```python
from build123d import *

# Parameters (mm, degrees)
F1_DEPTH = 25.4


with BuildPart() as f1:
    # F0 (on Top) → F1 (new body)
    with BuildSketch(Plane.XY):
        Polygon((123.5442494553, -9.8546108769), (0, 201.9159130813), (-122.2657690137, -9.8546108769), align=None)
        with BuildLine():
            Line((-4.8778088885, 178.2273002568), (0, 186.6759130813))
            Line((0, 186.6759130813), (4.8778088885, 178.2273002568))
            Line((4.8778088885, 178.2273002568), (107.7773886687, 0))
            Line((107.7773886687, 0), (14.1198557448, 0))
            ThreePointArc((14.1198557448, 0), (9.5256601261, -0.8879425347), (4.8778088885, -1.4288253328))
            ThreePointArc((4.8778088885, -1.4288253328), (-4.6759216184, -1.4443391195), (-14.1198557448, 0))
            Line((-14.1198557448, 0), (-107.7773886687, 0))
            Line((-107.7773886687, 0), (-4.8778088885, 178.2273002568))
        make_face(mode=Mode.SUBTRACT)
        with BuildLine():
            Line((-4.8778088885, 114.1285764535), (-4.8778088885, 122.8822744628))
            ThreePointArc((-4.8778088885, 122.8822744628), (-62.1710636846, 65.4026461834), (-14.1198557448, 0))
            Line((-14.1198557448, 0), (-4.8778088885, 0))
            Line((-4.8778088885, 0), (-4.8778088885, 7.3248726765))
            ThreePointArc((-4.8778088885, 7.3248726765), (-53.6241625079, 60.726724565), (-4.8778088885, 114.1285764535))
        make_face()
        with BuildLine():
            ThreePointArc((62.346655104, 60.726724565), (45.7778356363, 103.052782344), (4.8778088885, 122.8822744628))
            Line((4.8778088885, 122.8822744628), (4.8778088885, 114.1285764535))
            ThreePointArc((4.8778088885, 114.1285764535), (39.6050452669, 96.8790577412), (53.6241625079, 60.726724565))
            ThreePointArc((53.6241625079, 60.726724565), (39.6050452669, 24.5743913889), (4.8778088885, 7.3248726765))
            Line((4.8778088885, 7.3248726765), (4.8778088885, 0))
            Line((4.8778088885, 0), (14.1198557448, 0))
            ThreePointArc((14.1198557448, 0), (48.8233098985, 21.9531534991), (62.346655104, 60.726724565))
        make_face()
        with BuildLine():
            ThreePointArc((4.8778088885, 114.1285764535), (0, 114.3508870729), (-4.8778088885, 114.1285764535))
            Line((-4.8778088885, 114.1285764535), (-4.8778088885, 7.3248726765))
            ThreePointArc((-4.8778088885, 7.3248726765), (0, 7.1025620571), (4.8778088885, 7.3248726765))
            Line((4.8778088885, 7.3248726765), (4.8778088885, 114.1285764535))
        make_face()
        with BuildLine():
            Line((4.8778088885, 178.2273002568), (0, 186.6759130813))
            Line((0, 186.6759130813), (-4.8778088885, 178.2273002568))
            Line((-4.8778088885, 178.2273002568), (-4.8778088885, 122.8822744628))
            ThreePointArc((-4.8778088885, 122.8822744628), (0, 123.073379669), (4.8778088885, 122.8822744628))
            Line((4.8778088885, 122.8822744628), (4.8778088885, 178.2273002568))
        make_face()
        with BuildLine():
            ThreePointArc((4.8778088885, 122.8822744628), (0, 123.073379669), (-4.8778088885, 122.8822744628))
            Line((-4.8778088885, 122.8822744628), (-4.8778088885, 114.1285764535))
            ThreePointArc((-4.8778088885, 114.1285764535), (0, 114.3508870729), (4.8778088885, 114.1285764535))
            Line((4.8778088885, 114.1285764535), (4.8778088885, 122.8822744628))
        make_face()
        with BuildLine():
            Line((-4.8778088885, 7.3248726765), (-4.8778088885, 0))
            Line((-4.8778088885, 0), (4.8778088885, 0))
            Line((4.8778088885, 0), (4.8778088885, 7.3248726765))
            ThreePointArc((4.8778088885, 7.3248726765), (0, 7.1025620571), (-4.8778088885, 7.3248726765))
        make_face()
        with BuildLine():
            Line((-4.8778088885, 0), (-14.1198557448, 0))
            ThreePointArc((-14.1198557448, 0), (-4.6759216184, -1.4443391195), (4.8778088885, -1.4288253328))
            Line((4.8778088885, -1.4288253328), (4.8778088885, 0))
            Line((4.8778088885, 0), (-4.8778088885, 0))
        make_face()
        with BuildLine():
            ThreePointArc((4.8778088885, -1.4288253328), (9.5256601261, -0.8879425347), (14.1198557448, 0))
            Line((14.1198557448, 0), (4.8778088885, 0))
            Line((4.8778088885, 0), (4.8778088885, -1.4288253328))
        make_face()
    extrude(amount=F1_DEPTH)


solid = f1.part
```
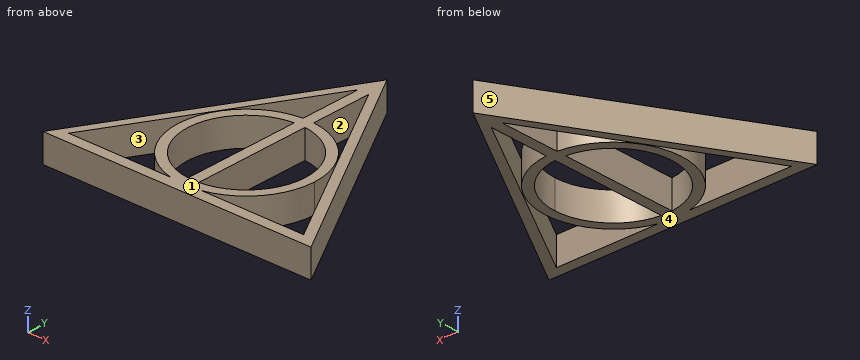
CAD build for the part. Positions are in the model's coordinates, mm. Face numbers are marked on the shaded views. A direction names the side the tool comes from. Round coordinates to 2 decimals unless told otherwise and drop trailing zeros. Order: outer loops, then holes, each group sorted by start corner. A loop starts at its lowest first (then second) coordinate and runs counter-clockwise, first axis right, second up. Notation, with made-up numbers: (61.5, 78.5) - (97.5, 78.5) arc R10 cw to (97.5, 85.5) - close; hole circle Ø5 at (76, 88.5). An arc over 180 degrees is marked (long way). Answer as CSV lines item,"result". Start each with the question number.
1. Saw through at C-C, the plane x = 74. Write the cut outline in (y, z), and give its area (3 significant figures).
2. Tool access for the marked faces 1 and 2: list every direction of +Z, -Z, +X, -X, +Y, -Y with a clear straight run to the whole face (end or side of a thin tool).
3. Saw through at A-A, the plane z = 10.25. Write the cut outline in (x, y), and give its area (3 significant figures).
4. Saw through at D-D, the plane x = -58. Write the cut outline in (y, z).
5. Drill centre lines: L1, parallel to Y at x = 34, z = 13.5; L2, parallel to X at y = 23.5, z = 16.75; L3, parallel to X at y = 150.5, z = 4 (3 decimals). Where is each one in solid material? Low to high. Write a range as [from, to].
6. Pull direction X, two halves, no side cores. Call the marked faces 3, 4 and 5: +X half, -X half, draft (parallel to the pull), parting line (faces both ways), or undercut.
7. Saw through at B-B, the plane y = 40. Write the cut outline in (x, z).
8. Pin check, flat tips, straight feed: pin 1 (7.5 mm diameter, centred on x = 65.5, z = 9.5, fed in from +Y); pin 2 (1.5 mm diameter, centred on x = 64.5, z = 20, fed in from +Y); pin 3 (7.5 mm diameter, centred on x = -60.5, z = 17.5, fed in from +Y). Stop position of each tip, or through.
Model answer:
1,outline,"(-9.85, 0) - (0, 0) - (0, 25.4) - (-9.85, 25.4) - close; (58.5, 0) - (75.07, 0) - (75.07, 25.4) - (58.5, 25.4) - close"
1,area,"671 mm²"
2,face 1,"+Z, +X, -X, +Y, -Y"
2,face 2,"+Z, -Z"
3,outline,"(-122.27, -9.85) - (123.54, -9.85) - (0, 201.92) - close; hole (-107.78, 0) - (-14.12, 0) arc R62.35 cw to (-4.88, 122.88) - (-4.88, 178.23) - close; hole (-4.88, 7.32) - (-4.88, 114.13) arc R53.62 ccw to start; hole (4.88, 7.32) arc R53.62 ccw to (4.88, 114.13) - close; hole (4.88, 122.88) arc R62.35 cw to (14.12, 0) - (107.78, 0) - (4.88, 178.23) - close"
3,area,"10,700 mm²"
4,outline,"(-9.85, 0) - (0, 0) - (0, 25.4) - (-9.85, 25.4) - close; (37.86, 0) - (83.6, 0) - (83.6, 25.4) - (37.86, 25.4) - close; (86.22, 0) - (101.46, 0) - (101.46, 25.4) - (86.22, 25.4) - close"
5,L1,"y = [-9.85, 0], [8.47, 19.26], [102.19, 112.99], [127.79, 143.64]"
5,L2,"x = [-103.01, -94.21], [-50.01, -38.6], [-4.88, 4.88], [38.6, 50.01], [94.21, 104.09]"
5,L3,"x = [-29.685, -20.886], [-4.878, 4.878], [20.886, 29.995]"
6,face 3,"undercut"
6,face 4,"draft"
6,face 5,"-X half"
7,outline,"(-93.48, 0) - (-84.68, 0) - (-84.68, 25.4) - (-93.48, 25.4) - close; (-58.8, 0) - (-49.46, 0) - (-49.46, 25.4) - (-58.8, 25.4) - close; (-4.88, 0) - (4.88, 0) - (4.88, 25.4) - (-4.88, 25.4) - close; (49.46, 0) - (58.8, 0) - (58.8, 25.4) - (49.46, 25.4) - close; (84.68, 0) - (94.46, 0) - (94.46, 25.4) - (84.68, 25.4) - close"
8,pin 1,"stops at y = 96.07"
8,pin 2,"stops at y = 92.64"
8,pin 3,"stops at y = 103.62"
